Check sheet for the drawn part. Datum: minimum x, y, z corner. Units: mm. A direction names the side the tool comes from. Round coordinates to 2 decimals unless told otherwise and drop trailing zeros. Write each loop counter-clockwise with the first axis right and the second up, starting at its lowest first coordinate (ties: lowest second). Pieces come first, ordered by that corner, then holes.
Item 1: Cross-section at D-D on y = 19.25. Enter the section's corners in (x, z), plus the area to 3 significant figures.
Item 2: Go/stop test with flat-tipped pins: pin 1 Ø10 at (x, y) = (69, 15.5) entering from -Z; pin 2 Ø12 at (x, y) = (92, 19.5) entering from -Z; pin 3 Ø15.5 at (x, z) = (31.25, 52.5) entering from +Y; pin 4 Ø10 at (x, y) = (50, 6) entering from +Z. Record where each tip stops, or that it passes through.
Item 3: Cross-section at B-B on x = 52.5. Enter the section's corners in (y, z), plus the area to 3 significant figures.
Item 4: Release check for a two-part mould opening along X. For the marked faces 1, 2 and 3 record: +X half, -X half, draft (parallel to the pull), parting line (faces both ways), or undercut.
Item 5: Material ranges on line 1 (Y direction, x = 52.5, z = 49.5); line 2 (X direction, y = 10, z = 50.5); line 3 (X direction, y = 13, z = 45), recorded low to high.
Item 6: Cross-section at A-A on z = 52.5. Enter the section's corners in (x, y), plus the area to 3 significant figures.
Item 7: Tool access check on the marked faces 4 and 5. Record the directions out of +Z, -Z, +X, -X, +Y, -Y that give a thin tool (end or side, any length) a straight path to the whole face; none if there is none.
Item 8: Cross-section at C-C on y = 8.5. Enter the section's corners in (x, z), plus the area to 3 significant figures.
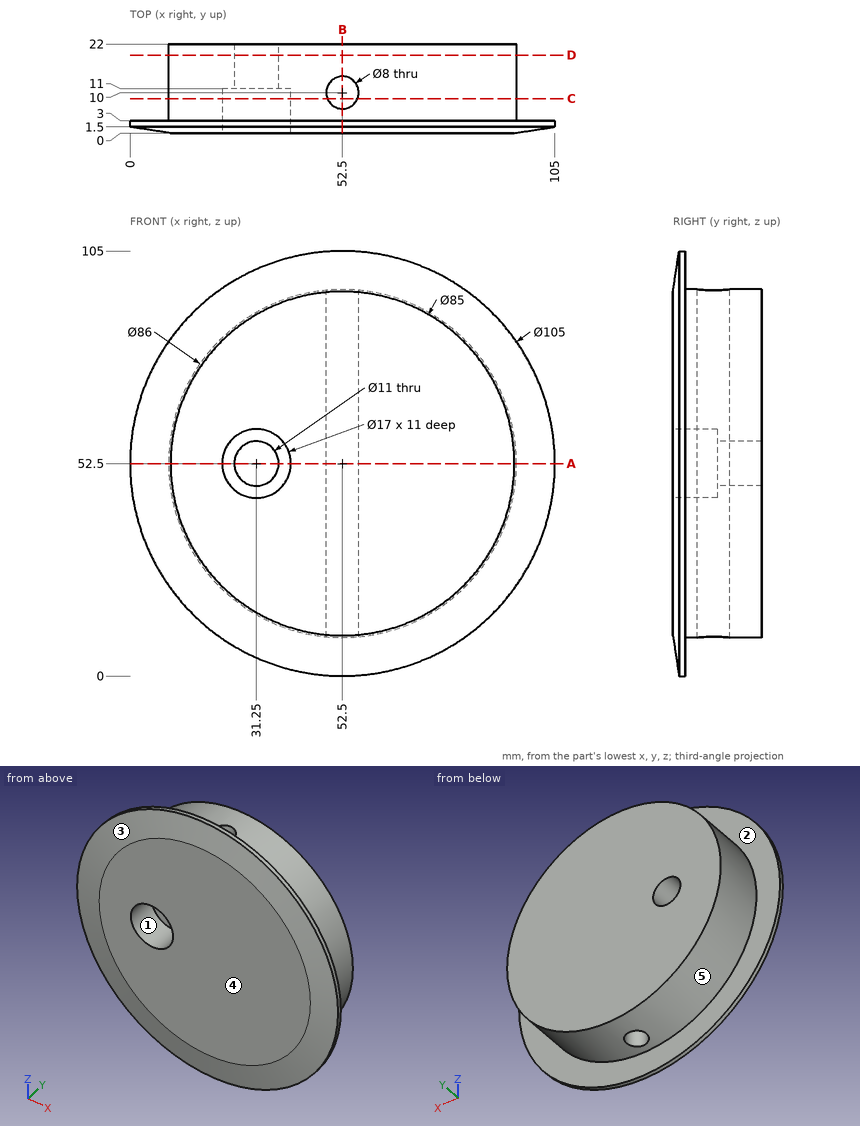
Response values:
1. outline: circle Ø86 at (52.5, 52.5); hole circle Ø11 at (31.25, 52.5)
1. area: 5,710 mm2
2. pin 1: stops at z = 11.07
2. pin 2: stops at z = 25.54
2. pin 3: stops at y = 22
2. pin 4: stops at z = 105
3. outline: (0, 10) - (1.5, 0) - (3, 0) - (3, 9.5) - (6, 9.5) - (6, 95.5) - (3, 95.5) - (3, 105) - (1.5, 105) - (0, 95) - close; (14, 9.5) - (22, 9.5) - (22, 95.5) - (14, 95.5) - close
3. area: 1,250 mm2
4. face 1: undercut
4. face 2: draft
4. face 3: parting line
5. line 1: y = 0 to 6, 14 to 22
5. line 2: x = 9.55 to 22.99, 39.51 to 48.5, 56.5 to 95.45
5. line 3: x = 10.16 to 49.85, 55.15 to 94.84
6. outline: (0, 1.5) - (10, 0) - (22.75, 0) - (22.75, 11) - (25.75, 11) - (25.75, 22) - (9.5, 22) - (9.5, 3) - (0, 3) - close; (36.75, 11) - (39.75, 11) - (39.75, 0) - (95, 0) - (105, 1.5) - (105, 3) - (95.5, 3) - (95.5, 22) - (36.75, 22) - close; hole circle Ø8 at (52.5, 10)
6. area: 1,580 mm2
7. face 4: +Z, -Z, +X, -X, -Y
7. face 5: +Y
8. outline: (48.79, 9.66) - (48.79, 95.34) arc R43 ccw to start; (56.21, 9.66) arc R43 ccw to (56.21, 95.34) - close; hole circle Ø17 at (31.25, 52.5)
8. area: 4,940 mm2
